Model file for the job. Use its own axes, mm. A direction names the side the tool comes from. Coordinates: 2 decimals unless noted, no trailing zeros. Write each loop counter-clockwise with the first axis right and the second up, starting at its lowest first coordinate (ties: lowest second). Pieces come first, ordered by that corner, then holes. Notation, with made-up numbers: M -38,-19.75 L -29,-19.75 A29 ccw -29,3.25 Z; hole C 24,-39 d10. An arc over 180 degrees is marked long. Put each result on its own line as item: value. Start each with the question number.
Q1. Drill centre lines: line 1 along Y through (x, z) = (0, 7.75); line 2 along Y through (x, z) = (0, 23.5); line 3 along Y through (x, z) = (-17, 21.25). Where is each one in solid material? Low to high.
Q2. Cut at C-C (x = 39.5). Write the cut outline in (y, z), then the cut area to 3 significant figures.
Q3. Cut at D-D (x = 6.5). Write the cut outline in (y, z).
Q4. Which spindle directions (+Z, -Z, +X, -X, +Y, -Y) get a long thin tool onto all of the face, cutting with end or side? Do faces 4 (the flat face through (-1, 1, 15)), 5 (the flat face through (49, -16, 30)). Say none if no direction does.
Q5. Cut at B-B (z = 12.75). Write the cut outline in (x, y), then the cut area to 3 significant figures.
Q6. Cut at A-A (y = 0). Write the cut outline in (x, z), then the cut area to 3 significant figures.
Q7. Pull direction Y, two halves, no side cores. Call faces 1 (the cylindrical face through (-9.764, 74.362, 14.79)), 2 (the cylindrical face through (6.791, -31.987, 7.395)), 3 (the flat face through (-1, 1, 0)): pulls with the +Y half, pulls with the -Y half, needs draft (parallel to the pull), parting line crosses it, or undercut.
Q8. Drop flat-ended pins along their axis: pin 1 (3 mm diameter, centred on y = 42, z = 11, fed in from -X); pin 2 (4 mm diameter, centred on y = -42.5, z = 18.5, fed in from +X); pin 3 (5 mm diameter, centred on x = 57, z = 11.5, fed in from +Y); pin 4 (4 mm diameter, centred on x = -57.5, y = 34.5, fed in from -Z). Give the stop position or say it passes through.
```python
from build123d import *

# Parameters (mm, degrees)
SKETCH1_R           = 75
SKETCH1_R_2         = 50
BOSS_EXTRUDE1_DEPTH = 30
BOSS_EXTRUDE2_DEPTH = 15


with BuildPart() as part:
    # Sketch1 → Boss-Extrude1 (new body)
    with BuildSketch(Plane.XY):
        Circle(SKETCH1_R)
        Circle(SKETCH1_R_2, mode=Mode.SUBTRACT)
    extrude(amount=BOSS_EXTRUDE1_DEPTH)

    # Sketch2 → Boss-Extrude2 (add)
    with BuildSketch(Plane(origin=(0, 0, 0), x_dir=(-1, 0, 0), z_dir=(0, 0, -1))):
        with BuildLine():
            ThreePointArc((-19.796645951, 5.331811511), (-30.803499375, 17.794882511), (-37.582797631, 32.977770122))
            ThreePointArc((-37.582797631, 32.977770122), (-43.211113504, 25.15550973), (-47.234297303, 16.398815759))
            ThreePointArc((-47.234297303, 16.398815759), (-32.262837592, -3.666350702), (-11.18835411, -17.180108765))
            ThreePointArc((-11.18835411, -17.180108765), (-26.44274376, -23.796947698), (-42.97744633, -25.552673186))
            ThreePointArc((-42.97744633, -25.552673186), (-37.277279866, -33.322731067), (-30.192401169, -39.854973487))
            ThreePointArc((-30.192401169, -39.854973487), (-6.482858375, -31.816746601), (12.881862833, -15.949702657))
            ThreePointArc((12.881862833, -15.949702657), (14.460984976, -32.502205015), (11.021275052, -48.770190652))
            ThreePointArc((11.021275052, -48.770190652), (20.17248754, -45.750090125), (28.57436718, -41.030543992))
            ThreePointArc((28.57436718, -41.030543992), (28.256210772, -15.997480106), (19.149783179, 7.322650414))
            ThreePointArc((19.149783179, 7.322650414), (35.380123986, 3.709480291), (49.788968911, -4.588962272))
            ThreePointArc((49.788968911, -4.588962272), (49.947214365, -2.296906009), (50, 0))
            ThreePointArc((50, 0), (49.460168644, 7.327463252), (47.852331292, 14.496702726))
            ThreePointArc((47.852331292, 14.496702726), (23.946157025, 21.929760162), (-1.046645951, 20.4753495))
            ThreePointArc((-1.046645951, 20.4753495), (7.405134174, 34.794789915), (19.75, 45.934055993))
            ThreePointArc((19.75, 45.934055993), (10.571343028, 48.869691083), (1, 49.989999))
            ThreePointArc((1, 49.989999), (-13.45667183, 29.550817252), (-19.796645951, 5.331811511))
        make_face()
    extrude(amount=-BOSS_EXTRUDE2_DEPTH)


solid = part.part
```
Computed values:
1. line 1: -75 to -50, -27.74 to 20.72, 22.91 to 48.99, 50 to 75
1. line 2: -75 to -50, 50 to 75
1. line 3: -73.05 to -47.02, 47.02 to 73.05
2. outline: M -63.76,0 L -25.6,0 L -25.6,15 L -30.66,15 L -30.66,30 L -63.76,30 Z; M 4.19,0 L 63.76,0 L 63.76,30 L 30.66,30 L 30.66,15 L 4.19,15 Z
2. area: 2,460 mm2
3. outline: M -74.72,0 L -49.58,0 L -49.58,30 L -74.72,30 Z; M -31.83,0 L 41.32,0 L 41.32,15 L -31.83,15 Z; M 49.58,0 L 74.72,0 L 74.72,30 L 49.58,30 Z
4. face 4: +Z
4. face 5: +Z, +X, -X, +Y, -Y
5. outline: C 0,0 d150; hole M -49.79,-4.59 A50 ccw -28.57,-41.03 A70 cw -19.15,7.32 A55 ccw Z; hole M -47.85,14.5 A70 cw 1.05,20.48 A55 ccw -19.75,45.93 A50 ccw Z; hole M -12.88,-15.95 A55 ccw -11.02,-48.77 A50 ccw 30.19,-39.85 A70 cw Z; hole M -1,49.99 A70 cw 19.8,5.33 A55 ccw 37.58,32.98 A50 ccw Z; hole M 11.19,-17.18 A55 ccw 42.98,-25.55 A50 ccw 47.23,16.4 A70 cw Z
5. area: 14,000 mm2
6. outline: M -75,0 L -43.09,0 L -43.09,15 L -50,15 L -50,30 L -75,30 Z; M -23.08,0 L 35.92,0 L 35.92,15 L -23.08,15 Z; M 50,0 L 75,0 L 75,30 L 50,30 Z
6. area: 2,490 mm2
7. face 1: parting line crosses it
7. face 2: undercut
7. face 3: needs draft
8. pin 1: x = -63.12
8. pin 2: x = 63.12
8. pin 3: y = 51.52
8. pin 4: z = 0
